```python
from build123d import *

# Parameters (mm, degrees)
BOSS_EXTRUDE1_DEPTH     = 45
CUT_EXTRUDE1_DEPTH      = 75.639131828
CUT_EXTRUDE1_DEPTH_BACK = 75.639131828
SKETCH3_R               = 1.35
SKETCH3_W               = 34.4
SKETCH3_H               = 34.4


with BuildPart() as part:
    # Sketch1 → Boss-Extrude1 (new body)
    with BuildSketch(Plane.XY):
        Polygon((0, 0), (44, 0), (44, 45), (39, 45), (39, 5), (5, 5), (5, 45), (0, 45), align=None)
    extrude(amount=BOSS_EXTRUDE1_DEPTH)

    # Sketch3 → Cut-Extrude1 (cut, two sides: drawn at the far end of the back side and taken through both)
    with BuildSketch(Plane(origin=(5, 0, 0), x_dir=(0, 0, -1), z_dir=(1, 0, 0)).offset(-CUT_EXTRUDE1_DEPTH_BACK)):
        with Locations((-37.2, 36.1)):
            Circle(SKETCH3_R)
        with Locations((-37.2, 14.1)):
            Circle(SKETCH3_R)
        with Locations((-31.9, 7.8)):
            Circle(SKETCH3_R)
        with Locations((-9.9, 7.8)):
            Circle(SKETCH3_R)
        with Locations((-17.2, 27.8)):
            Rectangle(SKETCH3_W, SKETCH3_H)
    extrude(amount=CUT_EXTRUDE1_DEPTH + CUT_EXTRUDE1_DEPTH_BACK, mode=Mode.SUBTRACT)


solid = part.part
```
CAD build for the part. Positions are in the model's coordinates, mm. A direction names the side the tool comes from. Round coordinates to 2 decimals unless told otherwise and drop trailing zeros. Order: outer loops, then holes, each group sorted by start corner. A loop starts at its lowest first (then second) coordinate and runs counter-clockwise, first axis right, second up.
Item 1: Saw through at A-A on x = 41.5. Write the cut outline in (y, z), then the cut area to 3 significant figures.
Item 2: Probe line 1 along Z through (x, y) = (3.25, 7.8); line 2 along Y through (x, z) = (42.7, 37.2); line 3 along X through (y, z) = (6, 9.5). List the from-to ranges inside material, lowest first.
Item 3: Tool access for faces 1 (the face through (5, 17, 36)), 2 (the face through (41.46, 36.16, 38.55)), 3 (the face through (41, 28, 34.4)): list every direction of +Z, -Z, +X, -X, +Y, -Y with a clear straight run to the whole face (end or side of a thin tool).
Item 4: Saw through at B-B on z = 37.2. Write the cut outline in (x, y), then the cut area to 3 significant figures.
Item 5: Saw through at D-D on y = 32. Write the cut outline in (x, z), then the cut area to 3 significant figures.
Item 6: Saw through at C-C on y = 14.1. Write the cut outline in (x, z), then the cut area to 3 significant figures.
Item 7: Pin check, flat tips, straight feed: pin 1 (3 mm diameter, centred on x = 10.5, z = 5.5, fed in from +Y); pin 2 (1.5 mm diameter, centred on x = 2, z = 11.5, fed in from +Y); pin 3 (2.5 mm diameter, centred on x = 2, y = 32.5, fed in from -Z). Stop position of each tip, or through.
Item 8: Mould opens along X. For faces 4 (the face through (44, 7, 27)), 5 (the face through (39, 19, 36)), 6 (the face through (22, 0, 22)) say: pulls with the +X half, pulls with the -X half, needs draft (parallel to the pull), parting line crosses it, or undercut.
Reported:
1. outline: (0, 0) - (10.6, 0) - (10.6, 34.4) - (45, 34.4) - (45, 45) - (0, 45) - close; hole circle Ø2.7 at (7.8, 9.9); hole circle Ø2.7 at (7.8, 31.9); hole circle Ø2.7 at (14.1, 37.2); hole circle Ø2.7 at (36.1, 37.2)
1. area: 819 mm2
2. line 1: z = 0 to 8.55, 11.25 to 30.55, 33.25 to 45
2. line 2: y = 0 to 12.75, 15.45 to 34.75, 37.45 to 45
2. line 3: x = 0 to 5, 39 to 44
3. face 1: +Z, -Z, +Y
3. face 2: +X, -X
3. face 3: -Z, +X, -X, +Y
4. outline: (0, 0) - (44, 0) - (44, 12.75) - (39, 12.75) - (39, 5) - (5, 5) - (5, 12.75) - (0, 12.75) - close; (0, 15.45) - (5, 15.45) - (5, 34.75) - (0, 34.75) - close; (0, 37.45) - (5, 37.45) - (5, 45) - (0, 45) - close; (39, 15.45) - (44, 15.45) - (44, 34.75) - (39, 34.75) - close; (39, 37.45) - (44, 37.45) - (44, 45) - (39, 45) - close
4. area: 566 mm2
5. outline: (0, 34.4) - (5, 34.4) - (5, 45) - (0, 45) - close; (39, 34.4) - (44, 34.4) - (44, 45) - (39, 45) - close
5. area: 106 mm2
6. outline: (0, 34.4) - (5, 34.4) - (5, 35.85) - (0, 35.85) - close; (0, 38.55) - (5, 38.55) - (5, 45) - (0, 45) - close; (39, 34.4) - (44, 34.4) - (44, 35.85) - (39, 35.85) - close; (39, 38.55) - (44, 38.55) - (44, 45) - (39, 45) - close
6. area: 79.0 mm2
7. pin 1: stops at y = 5
7. pin 2: stops at y = 10.6
7. pin 3: stops at z = 34.4
8. face 4: pulls with the +X half
8. face 5: undercut
8. face 6: needs draft
